```python
from build123d import *

# Parameters (mm, degrees)
F0_R     = 1.5
F1_DEPTH = 5
F2_SIZE  = 1.27


with BuildPart() as f1:
    # F0 (on Top) → F1 (new body)
    with BuildSketch(Plane.XY):
        with BuildLine():
            Line((-67.1149054365, 5.4482991469), (-60.9536656773, 5.4482991469))
            ThreePointArc((-60.9536656773, 5.4482991469), (-89.9189816406, -0.4755281134), (-60.6364599927, -4.5517008531))
            Line((-60.6364599927, -4.5517008531), (-66.5607646656, -4.5517008531))
            ThreePointArc((-66.5607646656, -4.5517008531), (-84.4382310461, -0.5270105536), (-67.1149054365, 5.4482991469))
        make_face()
        with BuildLine():
            ThreePointArc((-59.9291217554, 0), (-60.1874829455, 2.7718970869), (-60.9536656773, 5.4482991469))
            Line((-60.9536656773, 5.4482991469), (-67.1149054365, 5.4482991469))
            ThreePointArc((-67.1149054365, 5.4482991469), (-65.8409176364, 2.855485691), (-65.4028217554, 0))
            ThreePointArc((-65.4028217554, 0), (-65.69684554, -2.3483405013), (-66.5607646656, -4.5517008531))
            Line((-66.5607646656, -4.5517008531), (-60.6364599927, -4.5517008531))
            ThreePointArc((-60.6364599927, -4.5517008531), (-60.1070112283, -2.3031667351), (-59.9291217554, 0))
        make_face()
        with BuildLine():
            ThreePointArc((-11.6302119568, -4.5517008531), (-7.513293419, 0.6092107253), (-12.0040895417, 5.4482991469))
            Line((-12.0040895417, 5.4482991469), (-60.9536656773, 5.4482991469))
            ThreePointArc((-60.9536656773, 5.4482991469), (-60.1874829455, 2.7718970869), (-59.9291217554, 0))
            ThreePointArc((-59.9291217554, 0), (-60.1070112283, -2.3031667351), (-60.6364599927, -4.5517008531))
            Line((-60.6364599927, -4.5517008531), (-11.6302119568, -4.5517008531))
        make_face()
        with Locations((-50.4028217554, 0)):
            Circle(F0_R, mode=Mode.SUBTRACT)
        with Locations((-20.4028217554, 0)):
            Circle(F0_R, mode=Mode.SUBTRACT)
    extrude(amount=F1_DEPTH)

    # F2
    f2_edges = [f1.edges().sort_by_distance(p)[0] for p in [
        (-82.740738, -5.448299, 5),
        (-82.740738, -5.448299, 0),
    ]]
    chamfer(f2_edges, length=F2_SIZE)


solid = f1.part
```
The model under review builds one solid part; all positions refer to its coordinate system, in mm. A direction names the side the tool comes from. Round coordinates to 2 decimals unless told otherwise and drop trailing zeros. Order: outer loops, then holes, each group sorted by start corner. A loop starts at its lowest first (then second) coordinate and runs counter-clockwise, first axis right, second up. Notation, with made-up numbers: (-33, -4.5) -> (25, -4.5) arc R12 ccw to (25, 6.5) -> close; hole circle Ø11 at (19, 13). An arc over 180 degrees is marked (long way). One line per item, written item: value. Start each with the question number.
Q1. Take a section at A-A (z = 2.85). Write out the cut boundary in (x, y) (3 decimals).
Q2. Wall thickness on line 1 (Y direction, x = -13, z = 1.3); line 2 (Y direction, x = -50.5, z = 3.35); line 3 (X direction, y = 4, z = 3.65): over which ranges is each line inside the solid? List them lowest first.
Q3. Clearance check with flat-ended pins moving along their axes: pin 1 Ø8 at (x, y) = (-36, -3) entering from -Z; pin 2 Ø2.5 at (x, z) = (-30.5, 2.5) entering from +Y; pin 3 Ø11.5 at (x, y) = (-74.93, 0) entering from +Z (3 decimals); pin 4 Ø2 at (y, z) = (-11.5, 2.5) entering from -X. State where each tip first meets the part, or that it passes through.
Q4. Mouldability with a two-part tool opening along Y and no side actions: class faces 1 (the face through (-21.9, 0.1, 2.5)), 2 (the face through (-36, -4.552, 2)), 3 (the face through (-89.926, 0.113, 2.465)) as released by +Y, released by -Y, zero draft, split by the parting line, or undercut.
Q5. Take a section at B-B (x = -24). Write out the cut boundary in (y, z).
Q6. Machinability: for faces 4 (the face through (-7.51, 0.51, 2.46)), 5 (the face through (-36, 5.448, 2)), which of the approach directions +Z, -Z, +X, -X, +Y, -Y give a long, thin tool a straight path to every point of the face, cutting with its end or side? Answer none if there is none.
Reported:
1. outline: (-60.954, 5.448) arc R14.999 ccw (long way) to (-60.636, -4.552) -> (-11.63, -4.552) arc R5.06 ccw to (-12.004, 5.448) -> close; hole circle Ø19.05 at (-74.928, 0); hole circle Ø3 at (-50.403, 0); hole circle Ø3 at (-20.403, 0)
2. line 1: y = -4.55 to 5.45
2. line 2: y = -4.55 to -1.5, 1.5 to 5.45
2. line 3: x = -89.38 to -83.57, -66.28 to -8.99
3. pin 1: stops at z = 0
3. pin 2: stops at y = 5.45
3. pin 3: passes through
3. pin 4: stops at x = -85.64
4. face 1: undercut
4. face 2: released by -Y
4. face 3: split by the parting line
5. outline: (-4.55, 0) -> (5.45, 0) -> (5.45, 5) -> (-4.55, 5) -> close
6. face 4: +Z, -Z, +X
6. face 5: +Z, -Z, +X, +Y
